Source: CAD feature listing. Evaluate the final solid. Frame: model axes, mm. Face numbers are marked on the shaded views. A direction names the side the tool comes from. Give positions to 0.01 mm unless a question says otherwise; leave off trailing zeros. Order: outer loops, then holes, each group sorted by start corner. A loop starts at its lowest first (then second) coordinate and runs counter-clockwise, first axis right, second up.
1) Section D-D, the plane z = 22.5. Return loops of the section in (x, y), plus the area to 3 significant figures.
2) Draft query along Y for the marked faces 3, 4, 5 and 6. Return one class per face: released by +Y, released by -Y, zero draft, split by the parting line, or undercut.
3) Section A-A, the plane z = 17. Return loops of the section in (x, y).
4) Material intervals for line 1 (X direction, y = 13.75, z = 3.75); line 2 (X direction, y = 18.5, z = 17.25); line 3 (Y direction, x = -4.5, z = 12.5), sorted ascending.
5) Section B-B, the plane x = -9. Return loops of the section in (y, z).
6) First-contact query: P1, Ø6, axis at x = 0, z = 13, coming from the +Y side; P2, Ø0.6, axis at x = 10.5, z = 14.5, coming from the +Y side; P3, Ø1.4, axis at y = 12.5, z = 8.5, coming from the +X side. Flat tips, straight axial feed; report the tip coordinate or a pass-through.
7) Access query for the marked faces 1 and 2. Directions: +Z, -Z, +X, -X, +Y, -Y. A direction counts if a zero-diameter tool reaches every point of the face in a straight line with its end or side. Return the directions, or none.
8) Section C-C, the plane y = 15.75. Return loops of the section in (x, z), plus the area to 3 significant figures.
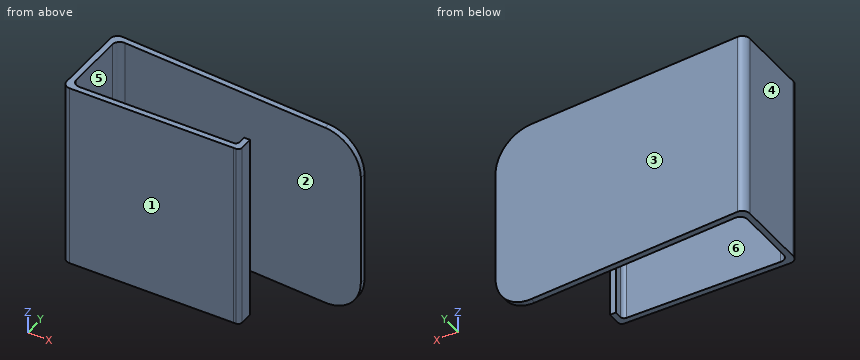
```python
from build123d import *

# Parameters (mm, degrees)
F1_DEPTH = 25
F2_R     = 5
F3_R     = 1
F4_R     = 0.5


# Not quite as in the source:
# - a feature names something its author has since deleted; it is built from what else it names


with BuildPart() as f1:
    # F0 (on Top) → F1 (new body)
    with BuildSketch(Plane.XY):
        Polygon((-12.9449461493, 23.2145217315), (-12.9449461493, 11.7507396201), (10.0550538507, 11.7507396201), (10.8550538507, 11.7466916821), (10.8550538507, 14.0507396201), (10.0550538507, 14.0507396201), (10.0550538507, 12.5507396201), (-12.1449461493, 12.5507396201), (-12.1449461493, 22.5507396201), (22.0030346708, 20.162880187), (22.0030346708, 20.9648337055), (-12.9449461493, 23.4086345881), align=None)
    extrude(amount=F1_DEPTH)

    # F2
    f2_edges = [f1.edges().sort_by_distance(p)[0] for p in [
        (22.003035, 20.563857, 25),
        (22.003035, 20.563857, 0),
    ]]
    fillet(f2_edges, radius=F2_R)

    # F3
    f3_edges = [f1.edges().sort_by_distance(p)[0] for p in [
        (-12.944946, 11.75074, 12.5),
        (-12.144946, 12.55074, 12.5),
        (-12.944946, 23.408635, 12.5),
        (-12.144946, 22.55074, 12.5),
    ]]
    fillet(f3_edges, radius=F3_R)

    # F4
    f4_edges = [f1.edges().sort_by_distance(p)[0] for p in [
        (10.855054, 11.746692, 12.5),
        (10.055054, 12.55074, 12.5),
    ]]
    fillet(f4_edges, radius=F4_R)


solid = f1.part
```
From the geometry:
1. outline: (-12.94, 12.75) arc R1 ccw to (-11.94, 11.75) - (10.06, 11.75) - (10.35, 11.75) arc R0.5 ccw to (10.86, 12.25) - (10.86, 14.05) - (10.06, 14.05) - (10.06, 13.05) arc R0.5 cw to (9.56, 12.55) - (-11.14, 12.55) arc R1 cw to (-12.14, 13.55) - (-12.14, 21.48) arc R1 cw to (-11.08, 22.48) - (21.33, 20.21) - (21.33, 21.01) - (-11.88, 23.33) arc R1 ccw to (-12.94, 22.34) - close
1. area: 55.8 mm2
2. face 3: released by +Y
2. face 4: zero draft
2. face 5: undercut
2. face 6: undercut
3. outline: (-12.94, 12.75) arc R1 ccw to (-11.94, 11.75) - (10.06, 11.75) - (10.35, 11.75) arc R0.5 ccw to (10.86, 12.25) - (10.86, 14.05) - (10.06, 14.05) - (10.06, 13.05) arc R0.5 cw to (9.56, 12.55) - (-11.14, 12.55) arc R1 cw to (-12.14, 13.55) - (-12.14, 21.48) arc R1 cw to (-11.08, 22.48) - (22, 20.16) - (22, 20.96) - (-11.88, 23.33) arc R1 ccw to (-12.94, 22.34) - close
4. line 1: x = -12.94 to -12.14, 10.06 to 10.86
4. line 2: x = -12.94 to -12.14
4. line 3: y = 11.75 to 12.55, 22.02 to 22.82
5. outline: (11.75, 0) - (12.55, 0) - (12.55, 25) - (11.75, 25) - close; (22.33, 0) - (23.13, 0) - (23.13, 25) - (22.33, 25) - close
6. P1: stops at y = 22.71
6. P2: stops at y = 21.79
6. P3: stops at x = 10.86
7. face 1: +Z, -Z, +X, -X, -Y
7. face 2: +Z, -Z
8. outline: (-12.94, 0) - (-12.14, 0) - (-12.14, 25) - (-12.94, 25) - close
8. area: 20.0 mm2
